```python
from build123d import *

# Parameters (mm, degrees)
F1_DEPTH = 3.5
F2_DEPTH = 150
F3_R     = 5
F4_R     = 1.5


with BuildPart() as f1:
    # F0 (on Front) → F1 (new body)
    with BuildSketch(Plane.XZ):
        with BuildLine():
            ThreePointArc((3.5, 8.5), (4.9644660941, 4.9644660941), (8.5, 3.5))
            Line((8.5, 3.5), (59.5, 3.5))
            ThreePointArc((59.5, 3.5), (63.0355339059, 4.9644660941), (64.5, 8.5))
            Line((64.5, 8.5), (64.5, 45))
            ThreePointArc((64.5, 45), (63.0355339059, 48.5355339059), (59.5, 50))
            Line((59.5, 50), (8.5, 50))
            ThreePointArc((8.5, 50), (4.9644660941, 48.5355339059), (3.5, 45))
            Line((3.5, 45), (3.5, 8.5))
        make_face()
    extrude(amount=-F1_DEPTH)

    # F0 (on Front) → F2 (join)
    with BuildSketch(Plane.XZ):
        with BuildLine():
            ThreePointArc((0, 5), (1.4644660941, 1.4644660941), (5, 0))
            Line((5, 0), (63, 0))
            ThreePointArc((63, 0), (66.5355339059, 1.4644660941), (68, 5))
            Line((68, 5), (68, 48.5))
            ThreePointArc((68, 48.5), (66.5355339059, 52.0355339059), (63, 53.5))
            Line((63, 53.5), (5, 53.5))
            ThreePointArc((5, 53.5), (1.4644660941, 52.0355339059), (0, 48.5))
            Line((0, 48.5), (0, 5))
        make_face()
        with BuildLine():
            Line((59.5, 3.5), (8.5, 3.5))
            ThreePointArc((8.5, 3.5), (4.9644660941, 4.9644660941), (3.5, 8.5))
            Line((3.5, 8.5), (3.5, 45))
            ThreePointArc((3.5, 45), (4.9644660941, 48.5355339059), (8.5, 50))
            Line((8.5, 50), (59.5, 50))
            ThreePointArc((59.5, 50), (63.0355339059, 48.5355339059), (64.5, 45))
            Line((64.5, 45), (64.5, 8.5))
            ThreePointArc((64.5, 8.5), (63.0355339059, 4.9644660941), (59.5, 3.5))
        make_face(mode=Mode.SUBTRACT)
    extrude(amount=-F2_DEPTH)

    # F3
    f3_edges = [f1.edges().sort_by_distance(p)[0] for p in [
        (34, 0, 53.5),
        (1.464466, 0, 52.035534),
        (0, 0, 26.75),
        (1.464466, 0, 1.464466),
        (34, 0, 0),
        (66.535534, 0, 1.464466),
        (68, 0, 26.75),
        (66.535534, 0, 52.035534),
    ]]
    fillet(f3_edges, radius=F3_R)

    # F4
    f4_edges = [f1.edges().sort_by_distance(p)[0] for p in [
        (34, 150, 53.5),
        (34, 150, 50),
        (1.464466, 150, 52.035534),
        (4.964466, 150, 48.535534),
        (0, 150, 26.75),
        (3.5, 150, 26.75),
        (1.464466, 150, 1.464466),
        (4.964466, 150, 4.964466),
        (34, 150, 3.5),
        (34, 150, 0),
        (66.535534, 150, 1.464466),
        (63.035534, 150, 4.964466),
        (68, 150, 26.75),
        (64.5, 150, 26.75),
        (63.035534, 150, 48.535534),
        (66.535534, 150, 52.035534),
    ]]
    fillet(f4_edges, radius=F4_R)


solid = f1.part
```
Part model, mm, in its own coordinate system. A direction names the side the tool comes from. Coordinates: 2 decimals unless noted, no trailing zeros. Order: outer loops, then holes, each group sorted by start corner. A loop starts at its lowest first (then second) coordinate and runs counter-clockwise, first axis right, second up. Notation, with made-up numbers: (52, 88) -> (56, 88) arc R8 cw to (56, 95) -> close; hole circle Ø10 at (89, -9). An arc over 180 degrees is marked (long way). Put each result on its own line as item: value. Start each with the question number.
(1) Band-saw the part on B-B (y = 118). Give the cut face in (x, z), then the cut area to 4 significant figures.
(2) Pin check, flat tip, straight feed: pin 1 Ø4 at (x, z) = (27.5, 26.5) entering from +Y. Stop position of the tip, or through.
(3) Probe line 1 along X through (y, z) = (12, 27.5); line 2 along Z through (x, y) = (13, 87); line 3 along Y through (x, z) = (25, 43.5). List the from-to ranges inside material, lowest first. Write a range as [from, to].
(4) Which spindle directions (+Z, -Z, +X, -X, +Y, -Y) get a long thin tool onto all of the face, cutting with end or side? Do faces 1 (the face through (34, 75, 50)), 2 (the face through (33.59, 1.43, 52)). Say none if no direction does.
(5) Mould opens along X. For faces 3 (the face through (63, 74.98, 48.57)), 4 (the face through (66, 76, 1)), 5 (the face through (4.93, 74.98, 48.5)), 6 (the face through (1.5, 75.75, 52.07)) say: pulls with the +X half, pulls with the -X half, needs draft (parallel to the pull), parting line crosses it, or undercut.
(6) Band-saw the part on C-C (x = 58). Give the cut face in (y, z), then the cut area to 3 significant figures.
(7) Band-saw the part on A-A (z = 30.5). Give the cut face in (x, y), then the cut area to 3 significant figures.
Determined:
1. outline: (0, 5) arc R5 ccw to (5, 0) -> (63, 0) arc R5 ccw to (68, 5) -> (68, 48.5) arc R5 ccw to (63, 53.5) -> (5, 53.5) arc R5 ccw to (0, 48.5) -> close; hole (3.5, 8.5) arc R5 ccw to (8.5, 3.5) -> (59.5, 3.5) arc R5 ccw to (64.5, 8.5) -> (64.5, 45) arc R5 ccw to (59.5, 50) -> (8.5, 50) arc R5 ccw to (3.5, 45) -> close
1. area: 801.5 mm²
2. pin 1: stops at y = 3.5
3. line 1: x = [0, 3.5], [64.5, 68]
3. line 2: z = [0, 3.5], [50, 53.5]
3. line 3: y = [0, 3.5]
4. face 1: +Y
4. face 2: +Z, +X, -X, -Y
5. face 3: undercut
5. face 4: pulls with the +X half
5. face 5: undercut
5. face 6: pulls with the -X half
6. outline: (0, 5) arc R5 ccw to (5, 0) -> (148.5, 0) arc R1.5 ccw to (150, 1.5) -> (150, 2) arc R1.5 ccw to (148.5, 3.5) -> (3.5, 3.5) -> (3.5, 50) -> (148.5, 50) arc R1.5 ccw to (150, 51.5) -> (150, 52) arc R1.5 ccw to (148.5, 53.5) -> (5, 53.5) arc R5 ccw to (0, 48.5) -> close
6. area: 1,200 mm²
7. outline: (0, 5) arc R5 ccw to (5, 0) -> (63, 0) arc R5 ccw to (68, 5) -> (68, 148.5) arc R1.5 ccw to (66.5, 150) -> (66, 150) arc R1.5 ccw to (64.5, 148.5) -> (64.5, 3.5) -> (3.5, 3.5) -> (3.5, 148.5) arc R1.5 ccw to (2, 150) -> (1.5, 150) arc R1.5 ccw to (0, 148.5) -> close
7. area: 1,250 mm²
